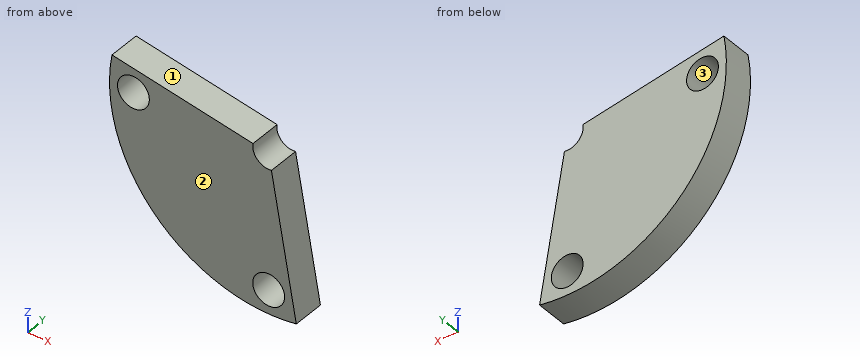
Autodesk Inventor part; units mm, degrees
ref_plane "YZ Plane" through (0, 0, 0) normal (1, 0, 0) x (0, 1, 0)
ref_plane "XZ Plane" through (0, 0, 0) normal (0, 1, 0) x (-1, 0, 0)
ref_plane "XY Plane" through (0, 0, 0) normal (0, 0, 1) x (1, 0, 0)
sketch "Sketch1" plane through (0, 0, 0) normal (0, 1, 0) x (-1, 0, 0)
  circle A0 centre (0, 0) radius 10
  line L0 (0, 0) -> (9.8481, 1.7365)
  line L1 (0, 0) -> (10, 0) construction
  line L2 (0, 0) -> (-1.7365, -9.8481)
  line L3 (0, 0) -> (10, 0) construction
  line L4 (10, 0) -> (8.5, 0)
  circle A1 centre (8.5, 0) radius 1
  line L5 (0, -10) -> (0, -8.5)
  circle A2 centre (0, -8.5) radius 1
  dimension "d0" = 20
  dimension "d1" = 10
  dimension "d2" = 100
  dimension "d3" = 1.5
  dimension "d4" = 2
  dimension "d5" = 1.5
  dimension "d6" = 2
extrude "Extrusion1" add sketch "Sketch1" along normal blind 2 contours A0 L2 L0 picked at (2.2606, -5.1604)
sketch "Sketch2" plane through (0, 2, 0) normal (0, 1, 0) x (1, 0, 0)
  line L0 (0, 0) -> (1.7365, 9.8481)
  circle A0 centre (0, 0) radius 1
  dimension "d9" = 2
extrude "Extrusion2" cut sketch "Sketch2" against normal blind 4
properties part number "bell_crank_small_v1"
Check sheet for the modelled part. Datum: model origin and axes. Units: mm. Face numbers are marked on the shaded views. Coordinates: 2 decimals unless noted, no trailing zeros. Loops run counter-clockwise (first coordinate to the right, second up) from the corner with the lowest first, then second, coordinate; pieces in that order, holes last.
1) Sectioned sample at A-A (z = 0). Record the boundary of the cut face in (x, y), and give its area (3 significant figures).
2) Sectioned sample at B-B (x = -0.75). Record the boundary of the cut face in (y, z).
3) Sectioned sample at C-C (y = 0.3). Record the boundary of the cut face in (x, z), and give its area (3 significant figures).
4) Material ranges on probe 1 along X at (y, z) = (1.1, -8.75); probe 2 along X at (y, z) = (1.5, -8.5), recorded low to high.
5) Gauge pin test, flat ends, axial feed: pin 1 (1 mm diameter, centred on y = 1, z = -1, fed in from -X); pin 2 (1 mm diameter, centred on x = -3, y = 0.5, fed in from +Z). Record the tip position at first contact, or that the pin passes through.
6) Release check for a two-part mould opening along X. For the marked faces 1, 2 and 3 record: released by +X, released by -X, zero draft, split by the parting line, or undercut.
7) Sectioned sample at D-D (x = -6). Record the boundary of the cut face in (y, z), and give its area (3 significant figures).
Check sheet entries:
1. outline: (-10, 0) - (-9.5, 0) - (-9.5, 2) - (-10, 2) - close; (-7.5, 0) - (-1, 0) - (-1, 2) - (-7.5, 2) - close
1. area: 14.0 mm2
2. outline: (0, -9.97) - (2, -9.97) - (2, -9.16) - (0, -9.16) - close; (0, -7.84) - (2, -7.84) - (2, -0.66) - (0, -0.66) - close
3. outline: (-9.85, 1.74) arc R10 ccw to (1.74, -9.85) - (0.17, -0.98) arc R1 cw to (-0.98, 0.17) - close; hole circle Ø2 at (-8.5, 0); hole circle Ø2 at (0, -8.5)
3. area: 88.8 mm2
4. probe 1: x = -4.84 to -0.97, 0.97 to 1.54
4. probe 2: x = -5.27 to -1, 1 to 1.5
5. pin 1: stops at x = -9.99
5. pin 2: stops at z = 0.62
6. face 1: released by +X
6. face 2: zero draft
6. face 3: undercut
7. outline: (0, -8) - (2, -8) - (2, 1.06) - (0, 1.06) - close
7. area: 18.1 mm2
